Print and shaded views of the part. All mm, measured from the part's lowest x, y and z. A direction names the side the tool comes from. Coordinates: 2 decimals unless noted, no trailing zeros. Loops run counter-clockwise (first coordinate to the right, second up) from the corner with the lowest first, then second, coordinate; pieces in that order, holes last. Notation, with made-up numbers: (-38.5, -21.75) -> (-6.5, -21.75) arc R25 cw to (-6.5, 0.25) -> close; hole circle Ø5 at (31, 33). An arc over 180 degrees is marked (long way). One line per question, with ' | ' between items. Start each with the question number.
1) 3-axis set-ups, long thin cutter, end or side, ignore diameter. For the marked faces 4 and 5: which of +Z, -Z, +X, -X, +Y, -Y reach the whole face in a straight line?
2) Drop flat-ended pins along their axis: pin 1 (0.5 mm diameter, centred on x = 4, z = 22.5, fed in from +Y); pin 2 (1.1 mm diameter, centred on y = 2, z = 22.5, fed in from -X); pin 3 (3 mm diameter, centred on x = 3.5, z = 9.5, fed in from +Y). Give the stop position or say it passes through.
3) Cut at D-D (x = 6.5). List the corners of the cut face in (y, z).
4) Two-plate mould, pull along Y, no slides. Class the marked faces 1, 2 and 3: released by +Y, released by -Y, zero draft, split by the parting line, or undercut.
5) Cut at C-C (z = 5). List the corners of the cut face in (x, y).
6) Probe L1, parallel to Z at x = 3.5, y = 1.95; L2, parallel to Y at x = 2, z = 6.5; L3, parallel to X at y = 4.1, z = 15.75. List the from-to ranges inside material, lowest first. Write a range as from..to.
7) Cut at A-A (x = 4.25). List the corners of the cut face in (y, z), plus the area to 3 significant figures.
8) Cut at B-B (y = 1.5). List the corners of the cut face in (x, z), plus the area to 3 significant figures.
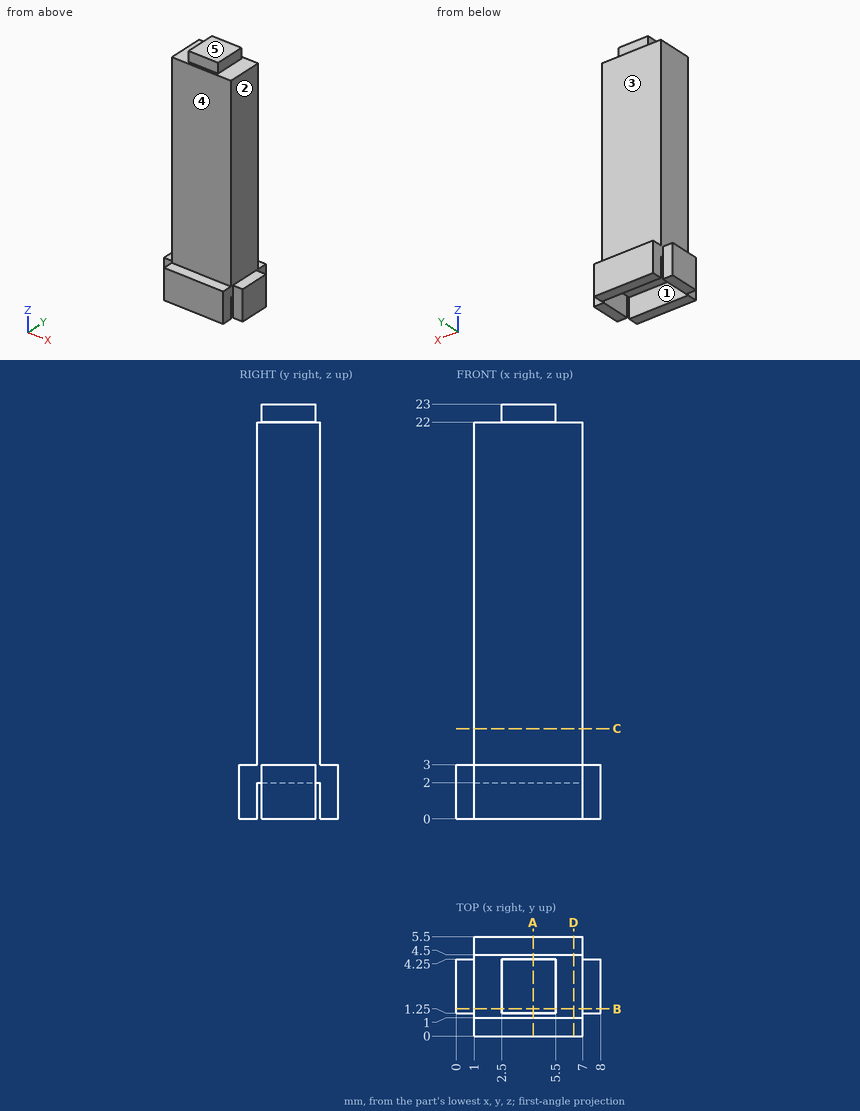
Reported:
1) face 4: +Z, +X, -X, -Y | face 5: +Z, +X, -X, +Y, -Y
2) pin 1: stops at y = 4.25 | pin 2: stops at x = 1 | pin 3: stops at y = 4.5
3) outline: (0, 0) -> (1, 0) -> (1, 2) -> (4.5, 2) -> (4.5, 0) -> (5.5, 0) -> (5.5, 3) -> (4.5, 3) -> (4.5, 22) -> (1, 22) -> (1, 3) -> (0, 3) -> close
4) face 1: undercut | face 2: zero draft | face 3: released by +Y
5) outline: (1, 1) -> (7, 1) -> (7, 4.5) -> (1, 4.5) -> close
6) L1: z = 2..23 | L2: y = 1..4.5 | L3: x = 1..7
7) outline: (0, 0) -> (1, 0) -> (1, 2) -> (4.5, 2) -> (4.5, 0) -> (5.5, 0) -> (5.5, 3) -> (4.5, 3) -> (4.5, 22) -> (4.25, 22) -> (4.25, 23) -> (1.25, 23) -> (1.25, 22) -> (1, 22) -> (1, 3) -> (0, 3) -> close | area: 79.0 mm²
8) outline: (0, 0) -> (1, 0) -> (1, 2) -> (7, 2) -> (7, 0) -> (8, 0) -> (8, 3) -> (7, 3) -> (7, 22) -> (5.5, 22) -> (5.5, 23) -> (2.5, 23) -> (2.5, 22) -> (1, 22) -> (1, 3) -> (0, 3) -> close | area: 129 mm²
